Build history of the part. All positions in model axes, mm. A direction names the side the tool comes from. Give positions to 0.01 mm unless a question says otherwise; leave off trailing zeros. Order: outer loops, then holes, each group sorted by start corner. A loop starts at its lowest first (then second) coordinate and runs counter-clockwise, first axis right, second up. Notation, with made-up numbers: (28, -25.5) - (70, -25.5) arc R30 ccw to (70, -3.5) - close; hole circle Ø11 at (60.5, -37.5). An arc over 180 degrees is marked (long way). One line per item, written item: value.
```python
from build123d import *

# Parameters (mm, degrees)
DODANIE_WYCI_GNI_CIE1_DEPTH      = 30
DODANIE_WYCI_GNI_CIE1_DEPTH_BACK = 30
SZKIC1_W                         = 60
SZKIC1_H                         = 60
ZAOKR_GLENIE1_R                  = 3
SZKIC2_W                         = 40
SZKIC2_H                         = 40
WYTNIJ_WYCI_GNI_CIE1_DEPTH       = 5
SZYK_KO_OWY1_COUNT               = 4
SZYK_KO_OWY2_COPY_1_SKETCH_W     = 40
SZYK_KO_OWY2_COPY_1_SKETCH_H     = 40
SZYK_KO_OWY2_COPY_1_DEPTH        = 5
SZYK_KO_OWY2_COPY_2_SKETCH_W     = 40
SZYK_KO_OWY2_COPY_2_SKETCH_H     = 40
SZYK_KO_OWY2_COPY_2_DEPTH        = 5
SZYK_KO_OWY2_COPY_3_SKETCH_W     = 40
SZYK_KO_OWY2_COPY_3_SKETCH_H     = 40
SZYK_KO_OWY2_COPY_3_DEPTH        = 5
SZYK_KO_OWY2_COPY_4_SKETCH_W     = 40
SZYK_KO_OWY2_COPY_4_SKETCH_H     = 40
SZYK_KO_OWY2_COPY_4_DEPTH        = 5
SZYK_KO_OWY2_COPY_5_SKETCH_W     = 40
SZYK_KO_OWY2_COPY_5_SKETCH_H     = 40
SZYK_KO_OWY2_COPY_5_DEPTH        = 5
SZYK_KO_OWY2_COPY_6_SKETCH_W     = 40
SZYK_KO_OWY2_COPY_6_SKETCH_H     = 40
SZYK_KO_OWY2_COPY_6_DEPTH        = 5
SZYK_KO_OWY2_COPY_7_SKETCH_W     = 40
SZYK_KO_OWY2_COPY_7_SKETCH_H     = 40
SZYK_KO_OWY2_COPY_7_DEPTH        = 5
SZYK_KO_OWY2_COPY_8_SKETCH_W     = 40
SZYK_KO_OWY2_COPY_8_SKETCH_H     = 40
SZYK_KO_OWY2_COPY_8_DEPTH        = 5
SZYK_KO_OWY2_COPY_9_SKETCH_W     = 40
SZYK_KO_OWY2_COPY_9_SKETCH_H     = 40
SZYK_KO_OWY2_COPY_9_DEPTH        = 5
SZYK_KO_OWY2_COPY_10_SKETCH_W    = 40
SZYK_KO_OWY2_COPY_10_SKETCH_H    = 40
SZYK_KO_OWY2_COPY_10_DEPTH       = 5
SZYK_KO_OWY2_COPY_11_SKETCH_W    = 40
SZYK_KO_OWY2_COPY_11_SKETCH_H    = 40
SZYK_KO_OWY2_COPY_11_DEPTH       = 5
SZYK_KO_OWY2_COPY_12_SKETCH_W    = 40
SZYK_KO_OWY2_COPY_12_SKETCH_H    = 40
SZYK_KO_OWY2_COPY_12_DEPTH       = 5


with BuildPart() as part:
    # Szkic1 → Dodanie-wyci_gni_cie1 (new, two sides: drawn at the far end of the back side and taken through both)
    with BuildSketch(Plane.XY.offset(-DODANIE_WYCI_GNI_CIE1_DEPTH_BACK)):
        Rectangle(SZKIC1_W, SZKIC1_H)
    extrude(amount=DODANIE_WYCI_GNI_CIE1_DEPTH + DODANIE_WYCI_GNI_CIE1_DEPTH_BACK)

    # Zaokr_glenie1
    zaokr_glenie1_edges = [part.edges().sort_by_distance(p)[0] for p in [
        (-30, 0, 30),
        (30, 0, -30),
        (0, -30, 30),
        (30, 0, 30),
        (0, 30, 30),
        (0, 30, -30),
        (-30, 0, -30),
        (-30, 30, 0),
        (30, 30, 0),
        (30, -30, 0),
        (-30, -30, 0),
        (0, -30, -30),
    ]]
    fillet(zaokr_glenie1_edges, radius=ZAOKR_GLENIE1_R)

    # Szkic2 → Wytnij-wyci_gni_cie1 (cut)
    with BuildSketch(Plane.XY.offset(30)):
        Rectangle(SZKIC2_W, SZKIC2_H)
    wytnij_wyci_gni_cie1 = extrude(amount=-WYTNIJ_WYCI_GNI_CIE1_DEPTH, mode=Mode.SUBTRACT)

    # Szyk ko_owy1: Wytnij-wyci_gni_cie1 ×4 about axis
    szyk_ko_owy1_axis = Axis((0, 0, 0), (1, 0, 0))
    for i in range(1, SZYK_KO_OWY1_COUNT):
        add(wytnij_wyci_gni_cie1.rotate(szyk_ko_owy1_axis, i * 360 / SZYK_KO_OWY1_COUNT), mode=Mode.SUBTRACT)

    # Szyk ko_owy2 copy 1 sketch → Szyk ko_owy2 copy 1 (cut)
    with BuildSketch(Plane.YZ.offset(30)):
        Rectangle(SZYK_KO_OWY2_COPY_1_SKETCH_W, SZYK_KO_OWY2_COPY_1_SKETCH_H)
    extrude(amount=-SZYK_KO_OWY2_COPY_1_DEPTH, mode=Mode.SUBTRACT)

    # Szyk ko_owy2 copy 2 sketch → Szyk ko_owy2 copy 2 (cut)
    with BuildSketch(Plane(origin=(0, 30, 0), x_dir=(-1, 0, 0), z_dir=(0, 1, 0))):
        Rectangle(SZYK_KO_OWY2_COPY_2_SKETCH_W, SZYK_KO_OWY2_COPY_2_SKETCH_H)
    extrude(amount=-SZYK_KO_OWY2_COPY_2_DEPTH, mode=Mode.SUBTRACT)

    # Szyk ko_owy2 copy 3 sketch → Szyk ko_owy2 copy 3 (cut)
    with BuildSketch(Plane(origin=(-30, 0, 0), x_dir=(0, -1, 0), z_dir=(-1, 0, 0))):
        Rectangle(SZYK_KO_OWY2_COPY_3_SKETCH_W, SZYK_KO_OWY2_COPY_3_SKETCH_H)
    extrude(amount=-SZYK_KO_OWY2_COPY_3_DEPTH, mode=Mode.SUBTRACT)

    # Szyk ko_owy2 copy 4 sketch → Szyk ko_owy2 copy 4 (cut)
    with BuildSketch(Plane.YX.offset(30)):
        Rectangle(SZYK_KO_OWY2_COPY_4_SKETCH_W, SZYK_KO_OWY2_COPY_4_SKETCH_H)
    extrude(amount=-SZYK_KO_OWY2_COPY_4_DEPTH, mode=Mode.SUBTRACT)

    # Szyk ko_owy2 copy 5 sketch → Szyk ko_owy2 copy 5 (cut)
    with BuildSketch(Plane(origin=(0, 0, -30), x_dir=(-1, 0, 0), z_dir=(0, 0, -1))):
        Rectangle(SZYK_KO_OWY2_COPY_5_SKETCH_W, SZYK_KO_OWY2_COPY_5_SKETCH_H)
    extrude(amount=-SZYK_KO_OWY2_COPY_5_DEPTH, mode=Mode.SUBTRACT)

    # Szyk ko_owy2 copy 6 sketch → Szyk ko_owy2 copy 6 (cut)
    with BuildSketch(Plane(origin=(0, 0, -30), x_dir=(0, -1, 0), z_dir=(0, 0, -1))):
        Rectangle(SZYK_KO_OWY2_COPY_6_SKETCH_W, SZYK_KO_OWY2_COPY_6_SKETCH_H)
    extrude(amount=-SZYK_KO_OWY2_COPY_6_DEPTH, mode=Mode.SUBTRACT)

    # Szyk ko_owy2 copy 7 sketch → Szyk ko_owy2 copy 7 (cut)
    with BuildSketch(Plane(origin=(-30, 0, 0), x_dir=(0, 1, 0), z_dir=(-1, 0, 0))):
        Rectangle(SZYK_KO_OWY2_COPY_7_SKETCH_W, SZYK_KO_OWY2_COPY_7_SKETCH_H)
    extrude(amount=-SZYK_KO_OWY2_COPY_7_DEPTH, mode=Mode.SUBTRACT)

    # Szyk ko_owy2 copy 8 sketch → Szyk ko_owy2 copy 8 (cut)
    with BuildSketch(Plane(origin=(0, -30, 0), x_dir=(-1, 0, 0), z_dir=(0, -1, 0))):
        Rectangle(SZYK_KO_OWY2_COPY_8_SKETCH_W, SZYK_KO_OWY2_COPY_8_SKETCH_H)
    extrude(amount=-SZYK_KO_OWY2_COPY_8_DEPTH, mode=Mode.SUBTRACT)

    # Szyk ko_owy2 copy 9 sketch → Szyk ko_owy2 copy 9 (cut)
    with BuildSketch(Plane(origin=(30, 0, 0), x_dir=(0, -1, 0), z_dir=(1, 0, 0))):
        Rectangle(SZYK_KO_OWY2_COPY_9_SKETCH_W, SZYK_KO_OWY2_COPY_9_SKETCH_H)
    extrude(amount=-SZYK_KO_OWY2_COPY_9_DEPTH, mode=Mode.SUBTRACT)

    # Szyk ko_owy2 copy 10 sketch → Szyk ko_owy2 copy 10 (cut)
    with BuildSketch(Plane(origin=(0, 0, 30), x_dir=(0, 1, 0), z_dir=(0, 0, 1))):
        Rectangle(SZYK_KO_OWY2_COPY_10_SKETCH_W, SZYK_KO_OWY2_COPY_10_SKETCH_H)
    extrude(amount=-SZYK_KO_OWY2_COPY_10_DEPTH, mode=Mode.SUBTRACT)

    # Szyk ko_owy2 copy 11 sketch → Szyk ko_owy2 copy 11 (cut)
    with BuildSketch(Plane(origin=(0, 0, 30), x_dir=(-1, 0, 0), z_dir=(0, 0, 1))):
        Rectangle(SZYK_KO_OWY2_COPY_11_SKETCH_W, SZYK_KO_OWY2_COPY_11_SKETCH_H)
    extrude(amount=-SZYK_KO_OWY2_COPY_11_DEPTH, mode=Mode.SUBTRACT)

    # Szyk ko_owy2 copy 12 sketch → Szyk ko_owy2 copy 12 (cut)
    with BuildSketch(Plane(origin=(0, 0, 30), x_dir=(0, -1, 0), z_dir=(0, 0, 1))):
        Rectangle(SZYK_KO_OWY2_COPY_12_SKETCH_W, SZYK_KO_OWY2_COPY_12_SKETCH_H)
    extrude(amount=-SZYK_KO_OWY2_COPY_12_DEPTH, mode=Mode.SUBTRACT)


solid = part.part
```
(1) Pull direction Y, two halves, no side cores. Call faces 1 (the face through (-30, 24, 0)), 2 (the face through (-20, 0, 28)), 3 (the face through (0, -25, 0)): +Y half, -Y half, draft (parallel to the pull), parting line (faces both ways), or undercut.
Completed:
face 1: draft
face 2: undercut
face 3: -Y half
(2) Drill centre lines: line 1 (X direction, y = -1, z = 26); line 2 (X direction, y = 10.5, z = 0). Where is each one in solid material? Low to high.
Completed:
line 1: -30 to -20, 20 to 30
line 2: -25 to 25
(3) Pin check, flat tips, straight feed: P1, Ø1.5, axis at x = 5, y = 5, coming from the -Z side; P2, Ø20, axis at x = 1.5, y = -5, coming from the +Z side; P3, Ø2.5, axis at x = -27.5, y = -10, coming from the +Z side; P4, Ø6, axis at y = -7, z = 8.5, coming from the -X side. Stop position of each tip, or through.
Completed:
P1: z = -25
P2: z = 25
P3: z = 30
P4: x = -25
(4) 3-axis set-ups, long thin cutter, end or side, ignore diameter. For faces 4 (the face through (0, -28, -20)), 5 (the face through (-28, 0, -20)), 6 (the face through (0, 0, 25)), 7 (the face through (-20, 0, -28)): which of +Z, -Z, +X, -X, +Y, -Y reach the whole face in a straight line?
Completed:
face 4: -Y
face 5: -X
face 6: +Z
face 7: -Z
(5) Slice it at A-A, the plane y = -7. Give the cut face in (x, z), and give its area (3 significant figures).
Completed:
outline: (-30, -27) arc R3 ccw to (-27, -30) - (-20, -30) - (-20, -25) - (20, -25) - (20, -30) - (27, -30) arc R3 ccw to (30, -27) - (30, -20) - (25, -20) - (25, 20) - (30, 20) - (30, 27) arc R3 ccw to (27, 30) - (20, 30) - (20, 25) - (-20, 25) - (-20, 30) - (-27, 30) arc R3 ccw to (-30, 27) - (-30, 20) - (-25, 20) - (-25, -20) - (-30, -20) - close
area: 2,790 mm²
